Here's how the part is built. I have some questions about the finished solid (model axes, mm). A direction names the side the tool comes from. Give positions to 0.01 mm unless a question says otherwise; leave off trailing zeros. Loops run counter-clockwise (first coordinate to the right, second up) from the corner with the lowest first, then second, coordinate; pieces in that order, holes last.
Q1. Will these pins go through, and if not, where does the flat tip stop? P1, Ø1.1, axis at x = -9, y = 16.5, coming from the -Z side; P2, Ø1.5, axis at y = 30, z = 11.5, coming from the -X side; P3, Ø2, axis at y = 14, z = 17.5, coming from the +X side; P4, Ø6, axis at x = -2.5, y = 19, coming from the +Z side.
Q2. If we section it at B-B (y = 18): Please give me the cut outline in (x, z).
Q3. If we section it at D-D (z = 28.5): Please give me the cut outline in (x, y).
Q4. If we section it at C-C (y = 28): Please give me the cut outline in (x, z), plus the area to 3 significant figures.
Q5. If we section it at A-A (x = -5.5): Please give me the cut outline in (y, z), plus the area to 3 significant figures.
Q6. We'd pull the mould along Z, two halves only. Please class faces 5 (the face through (-1.49, 0.57, 0.6)), 6 (the face through (0, 17, 30)), 7 (the face through (-8, 22.56, 30.5)): +Z half, -Z half, draft (parallel to the pull), parting line (faces both ways), or undercut.
Q7. For faces 1 (the face through (-0.5, 18, 26.4)), 2 (the face through (0, 19.5, 31)), 3 (the face through (-8, 22, 31)), 4 (the face through (-8, 19.02, 30.5)), which set-ups out of +Z, -Z, +X, -X, +Y, -Y let a thin tool reach every point of the face, with its end or its side?
Q8. I need wall thicknesses on line 1 (X direction, y = 14, z = 15.5); line 2 (X direction, y = 6, z = 2.5); line 3 (Z direction, x = -8, y = 22.5). Which ranges of each line are inside material? Lowest first, please.
from build123d import *

# Parameters (mm, degrees)
BOX003001_W           = 2.54
BOX003001_H           = 2.54
BOX003001_DEPTH       = 2.54
BOX002001_W           = 12
BOX002001_H           = 1
BOX002001_DEPTH       = 1
BOX003001001_W        = 2.54
BOX003001001_H        = 2.54
BOX003001001_DEPTH    = 2.54
BOX002001001_W        = 12
BOX002001001_H        = 1
BOX002001001_DEPTH    = 1
BOX003001001001_W     = 2.54
BOX003001001001_H     = 2.54
BOX003001001001_DEPTH = 2.54
BOX002001001001_W     = 12
BOX002001001001_H     = 1
BOX002001001001_DEPTH = 1
BOX003_W              = 2.54
BOX003_H              = 2.54
BOX003_DEPTH          = 2.54
BOX002_W              = 12
BOX002_H              = 1
BOX002_DEPTH          = 1
BOX_W                 = 1
BOX_H                 = 35.5
BOX_DEPTH             = 32
FILLET_R              = 2
FILLET001_R           = 2
FILLET002_R           = 2
FILLET003_R           = 2
BOX001_W              = 1
BOX001_H              = 35.5
BOX001_DEPTH          = 23


with BuildPart() as housing001:
    # Box003001 → Box003001 (new body)
    with BuildSketch(Plane(origin=(-5, 13.1, 29.3), x_dir=(1, 0, 0), z_dir=(0, 0, 1))):
        with Locations((1.27, 1.27)):
            Rectangle(BOX003001_W, BOX003001_H)
    extrude(amount=BOX003001_DEPTH)


with BuildPart() as pin003:
    # Box002001 → Box002001 (new body)
    with BuildSketch(Plane(origin=(-11, 13.94, 30), x_dir=(1, 0, 0), z_dir=(0, 0, 1))):
        with Locations((6, 0.5)):
            Rectangle(BOX002001_W, BOX002001_H)
    extrude(amount=BOX002001_DEPTH)

    # Fusion001: union Housing001
    add(housing001.part)


with BuildPart() as pin003_1:
    # Fusion001 placement: moved
    add(pin003.part.moved(Location((0, 2.54, 0))))


with BuildPart() as housing002:
    # Box003001001 → Box003001001 (new body)
    with BuildSketch(Plane(origin=(-5, 13.1, 29.3), x_dir=(1, 0, 0), z_dir=(0, 0, 1))):
        with Locations((1.27, 1.27)):
            Rectangle(BOX003001001_W, BOX003001001_H)
    extrude(amount=BOX003001001_DEPTH)


with BuildPart() as pin004:
    # Box002001001 → Box002001001 (new body)
    with BuildSketch(Plane(origin=(-11, 13.94, 30), x_dir=(1, 0, 0), z_dir=(0, 0, 1))):
        with Locations((6, 0.5)):
            Rectangle(BOX002001001_W, BOX002001001_H)
    extrude(amount=BOX002001001_DEPTH)

    # Fusion001001: union Housing002
    add(housing002.part)


with BuildPart() as pin004_1:
    # Fusion001001 placement: moved
    add(pin004.part.moved(Location((0, 5.08, 0))))


with BuildPart() as housing003:
    # Box003001001001 → Box003001001001 (new body)
    with BuildSketch(Plane(origin=(-5, 13.1, 29.3), x_dir=(1, 0, 0), z_dir=(0, 0, 1))):
        with Locations((1.27, 1.27)):
            Rectangle(BOX003001001001_W, BOX003001001001_H)
    extrude(amount=BOX003001001001_DEPTH)


with BuildPart() as pin006:
    # Box002001001001 → Box002001001001 (new body)
    with BuildSketch(Plane(origin=(-11, 13.94, 30), x_dir=(1, 0, 0), z_dir=(0, 0, 1))):
        with Locations((6, 0.5)):
            Rectangle(BOX002001001001_W, BOX002001001001_H)
    extrude(amount=BOX002001001001_DEPTH)

    # Fusion001001001: union Housing003
    add(housing003.part)


with BuildPart() as pin006_1:
    # Fusion001001001 placement: moved
    add(pin006.part.moved(Location((0, 7.62, 0))))


with BuildPart() as housing:
    # Box003 → Box003 (new body)
    with BuildSketch(Plane(origin=(-5, 13.1, 29.3), x_dir=(1, 0, 0), z_dir=(0, 0, 1))):
        with Locations((1.27, 1.27)):
            Rectangle(BOX003_W, BOX003_H)
    extrude(amount=BOX003_DEPTH)


with BuildPart() as pins:
    # Box002 → Box002 (new body)
    with BuildSketch(Plane(origin=(-11, 13.94, 30), x_dir=(1, 0, 0), z_dir=(0, 0, 1))):
        with Locations((6, 0.5)):
            Rectangle(BOX002_W, BOX002_H)
    extrude(amount=BOX002_DEPTH)

    # Fusion: union Housing
    add(housing.part)

    # Fusion001001002: union Pin003, Pin004, Pin006
    add(pin003_1.part)
    add(pin004_1.part)
    add(pin006_1.part)


with BuildPart() as pcb:
    # Box → Box (new body)
    with BuildSketch(Plane(origin=(-2, 0, 0), x_dir=(1, 0, 0), z_dir=(0, 0, 1))):
        with Locations((0.5, 17.75)):
            Rectangle(BOX_W, BOX_H)
    extrude(amount=BOX_DEPTH)

    # Fillet
    fillet_edges = [pcb.edges().sort_by_distance(p)[0] for p in [
        (-1.5, 0, 32),
    ]]
    fillet(fillet_edges, radius=FILLET_R)

    # Fillet001
    fillet001_edges = [pcb.edges().sort_by_distance(p)[0] for p in [
        (-1.5, 35.5, 32),
    ]]
    fillet(fillet001_edges, radius=FILLET001_R)

    # Fillet002
    fillet002_edges = [pcb.edges().sort_by_distance(p)[0] for p in [
        (-1.5, 0, 0),
    ]]
    fillet(fillet002_edges, radius=FILLET002_R)

    # Fillet003
    fillet003_edges = [pcb.edges().sort_by_distance(p)[0] for p in [
        (-1.5, 35.5, 0),
    ]]
    fillet(fillet003_edges, radius=FILLET003_R)


with BuildPart() as lcd:
    # Box001 → Box001 (new body)
    with BuildSketch(Plane(origin=(-1, 0, 3.4), x_dir=(1, 0, 0), z_dir=(0, 0, 1))):
        with Locations((0.5, 17.75)):
            Rectangle(BOX001_W, BOX001_H)
    extrude(amount=BOX001_DEPTH)

    # Fusion001001003: union Pins, Pcb
    add(pins.part)
    add(pcb.part)


solid = lcd.part
Check sheet entries:
1. P1: stops at z = 30
1. P2: stops at x = -2
1. P3: stops at x = 0
1. P4: stops at z = 32
2. outline: (-5, 29.3) - (-2.46, 29.3) - (-2.46, 31.84) - (-5, 31.84) - close; (-2, 0) - (-1, 0) - (-1, 3.4) - (0, 3.4) - (0, 26.4) - (-1, 26.4) - (-1, 32) - (-2, 32) - close
3. outline: (-2, 0) - (-1, 0) - (-1, 35.5) - (-2, 35.5) - close
4. outline: (-2, 0) - (-1, 0) - (-1, 3.4) - (0, 3.4) - (0, 26.4) - (-1, 26.4) - (-1, 32) - (-2, 32) - close
4. area: 55.0 mm2
5. outline: (13.94, 30) - (14.94, 30) - (14.94, 31) - (13.94, 31) - close; (16.48, 30) - (17.48, 30) - (17.48, 31) - (16.48, 31) - close; (19.02, 30) - (20.02, 30) - (20.02, 31) - (19.02, 31) - close; (21.56, 30) - (22.56, 30) - (22.56, 31) - (21.56, 31) - close
5. area: 4.00 mm2
6. face 5: -Z half
6. face 6: undercut
6. face 7: draft
7. face 1: +X, +Y, -Y
7. face 2: +Z, +X, +Y, -Y
7. face 3: +Z, -X, +Y, -Y
7. face 4: +Z, -Z, -X
8. line 1: x = -2 to 0
8. line 2: x = -2 to -1
8. line 3: z = 30 to 31
